Can you work these out from the drawing? Everything is in mm from the part's minimum corner. Coordinates: 2 decimals unless noted, no trailing zeros. Loops run counter-clockwise (first coordinate to the right, second up) from the corner with the lowest first, then second, coordinate; pieces in that order, holes last.
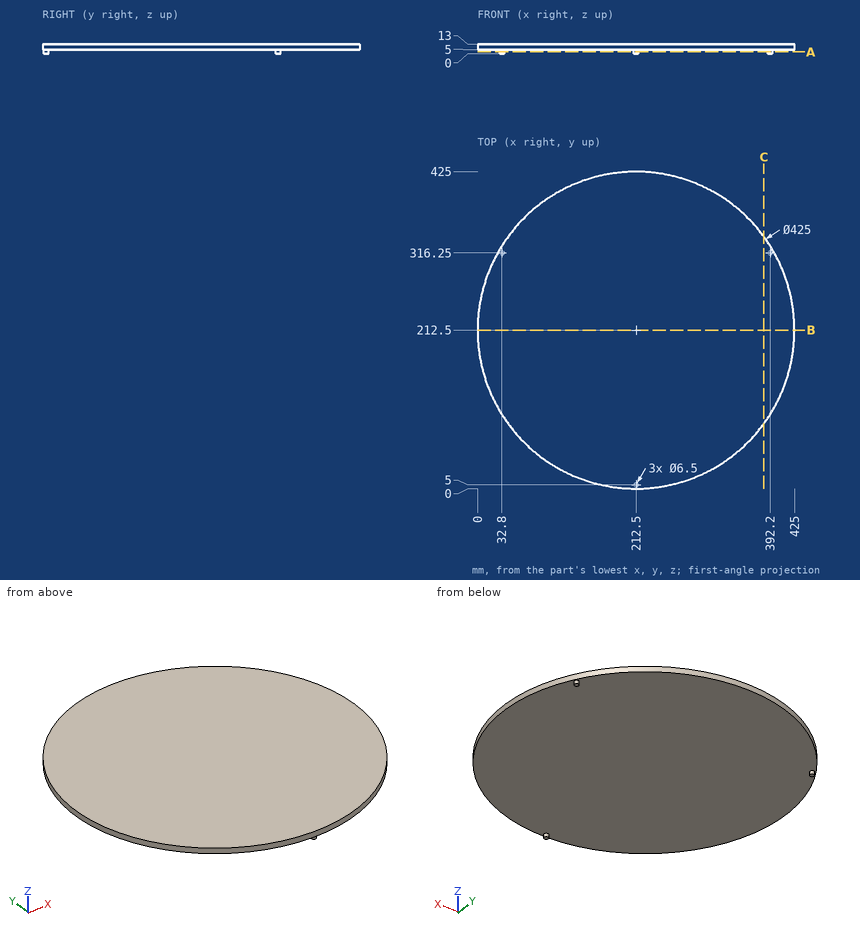
1) Imagine slicing it at A-A on z = 2.5. List the corners of the cut face in (x, y) for me.
2) Imagine slicing it at C-C on x = 384. List the corners of the cut face in (y, z) for me (1 decimal), plus the area to 3 significant figures.
3) Imagine slicing it at B-B on y = 212.5. List the corners of the cut face in (x, z) for me, plus the area to 3 significant figures.
4) If I drill on L1, parallel to Z at x = 299, y = 18.5; L2, parallel to X at y = 35.5, z = 11.5; L3, parallel to Y at x = 275, z = 9.25, over which ranges is the centre line in solid material (lowest first)?
5) Will these pins go through, and if not, where does the flat tip stop? pin 1 (1 mm diameter, centred on y = 138.5, z = 9.5, fed in from +X); pin 2 (1 mm diameter, centred on x = 188.5, y = 378, fed in from -Z); pin 3 (1.5 mm diameter, centred on x = 126.5, z = 8, fed in from -Y).
Solved:
1. outline: circle Ø6.5 at (32.8, 316.25); circle Ø6.5 at (212.5, 5); circle Ø6.5 at (392.2, 316.25)
2. outline: (87, 5) - (338, 5) - (338, 13) - (87, 13) - close
2. area: 2,010 mm2
3. outline: (0, 5) - (425, 5) - (425, 13) - (0, 13) - close
3. area: 3,400 mm2
4. L1: z = 5 to 13
4. L2: x = 94.91 to 330.09
4. L3: y = 9.4 to 415.6
5. pin 1: stops at x = 411.88
5. pin 2: stops at z = 5
5. pin 3: stops at y = 17.85
